Here's how the part is built. I have some questions about the finished solid (model axes, mm). Round coordinates to 2 decimals unless told otherwise and drop trailing zeros. Loops run counter-clockwise (first coordinate to the right, second up) from the corner with the lowest first, then second, coordinate; pieces in that order, holes last. Notation, with made-up numbers: (32, 34) - (52, 34) arc R25 ccw to (52, 53) - close; hole circle Ø8 at (10.5, -9.75). An arc over 180 degrees is marked (long way). Answer as a JSON object with one key per item and string values. Group by question number.
1) I want a section at C-C, the plane y = -2.25. Please give me the cut outline in (x, z).
2) I want a section at B-B, the plane z = 0. Please give me the cut outline in (x, y).
3) Will this pin go through, and if not, where does the flat tip stop? P1, Ø1, axis at x = -2.5, z = -7.5, coming from the +Y side.
4) If I drill on line 1 along Z through (x, y) = (0, -3.75); line 2 along X through (y, z) = (-3, 1); line 3 along X through (y, z) = (-10.5, 5.5), over which ranges is the centre line in solid material (lowest first)? Write a range as [from, to].
5) I want a section at A-A, the plane x = 0. Please give me the cut outline in (y, z).
6) If we mould it in two halves opening along X, with no side actions, what happens to faces 1 (the face through (-6, 0, 3)), 2 (the face through (12.051, -6.261, -12.023)), 3 (the face through (5.945, -6.439, 1.872)), 4 (the face through (-12.023, -6.261, -12.051))? For each: pulls with the +X half, pulls with the -X half, needs draft (parallel to the pull), parting line crosses it, or undercut.
from build123d import *

# Parameters (mm, degrees)
F0_W     = 26.0732
F0_H     = 26.0732
F1_DEPTH = 12.7
F2_R     = 6.23275
F3_DEPTH = 12.701
F4_SIZE  = 2


with BuildPart() as f1:
    # F0 (on Front) → F1 (new body)
    with BuildSketch(Plane.XZ):
        Rectangle(F0_W, F0_H)
    extrude(amount=F1_DEPTH)

    # F2 (on face) → F3 (cut, through all)
    with BuildSketch(Plane.XZ.offset(12.7)):
        Circle(F2_R)
    extrude(amount=-F3_DEPTH, mode=Mode.SUBTRACT)

    # F4
    f4_edges = [f1.edges().sort_by_distance(p)[0] for p in [
        (13.0366, -6.35, -13.0366),
        (13.0366, -6.35, 13.0366),
        (-13.0366, -6.35, -13.0366),
        (-13.0366, -6.35, 13.0366),
    ]]
    chamfer(f4_edges, length=F4_SIZE)


solid = f1.part
Outcome:
{
 "1": {"outline": "(-13.04, -11.04) - (-11.04, -13.04) - (11.04, -13.04) - (13.04, -11.04) - (13.04, 11.04) - (11.04, 13.04) - (-11.04, 13.04) - (-13.04, 11.04) - close; hole circle Ø12.47 at (0, 0)"},
 "2": {"outline": "(-13.04, -12.7) - (-6.23, -12.7) - (-6.23, 0) - (-13.04, 0) - close; (6.23, -12.7) - (13.04, -12.7) - (13.04, 0) - (6.23, 0) - close"},
 "3": {"P1": "y = 0"},
 "4": {"line 1": "[-13.04, -6.23], [6.23, 13.04]", "line 2": "[-13.04, -6.15], [6.15, 13.04]", "line 3": "[-13.04, -2.93], [2.93, 13.04]"},
 "5": {"outline": "(-12.7, -13.04) - (0, -13.04) - (0, -6.23) - (-12.7, -6.23) - close; (-12.7, 6.23) - (0, 6.23) - (0, 13.04) - (-12.7, 13.04) - close"},
 "6": {"face 1": "needs draft", "face 2": "pulls with the +X half", "face 3": "undercut", "face 4": "pulls with the -X half"}
}
